For this review, take the finished solid that the model builds, in its own axes (mm). Face numbers are marked on the shaded views. A direction names the side the tool comes from. Round coordinates to 2 decimals unless told otherwise and drop trailing zeros. Write each loop counter-clockwise with the first axis right and the second up, starting at its lowest first coordinate (ties: lowest second). Pieces come first, ordered by that corner, then holes.
from build123d import *

# Parameters (mm, degrees)
SKETCH1_W                  = 30
SKETCH1_H                  = 9.5
CUT_EXTRUDE1_DEPTH         = 3.5
SKETCH3_R                  = 17.4
BOSS_EXTRUDE1_DEPTH        = 4
SKETCH4_R                  = 10
BOSS_EXTRUDE2_DEPTH        = 16
CUT_EXTRUDE2_DEPTH         = 50.759421218
SKETCH6_W                  = 4
SKETCH6_H                  = 26
F_4_CLEARANCE_HOLE1_D      = 3.3
F_2_CLEARANCE_HOLE1_D      = 2.5
F_2_CLEARANCE_HOLE1_DEPTH  = 12
F_2_CLEARANCE_HOLE2_REACH  = 54.582
F_2_CLEARANCE_HOLE2_BORE_R = 1.25
F_2_CLEARANCE_HOLE3_D      = 2.5
F_2_CLEARANCE_HOLE3_DEPTH  = 40
FILLET1_R                  = 3


with BuildPart() as part:
    # Sketch1 → Revolve1 (revolve)
    with BuildSketch(Plane.XZ, mode=Mode.PRIVATE) as revolve1_sk:
        with Locations((15, 5.25)):
            Rectangle(SKETCH1_W, SKETCH1_H)
    revolve(revolve1_sk.sketch.rotate(Axis((0, 0, 10), (0, 0, -1)), 180), axis=Axis((0, 0, 10), (0, 0, -1)))

    # Sketch2 → Cut-Extrude1 (cut)
    with BuildSketch(Plane(origin=(0, 0, 0.5), x_dir=(-1, 0, 0), z_dir=(0, 0, -1))):
        with BuildLine():
            ThreePointArc((1.901854596, -26.932934283), (6.318658968, -26.250229501), (10.562335147, -24.848281153))
            ThreePointArc((10.562335147, -24.848281153), (13.103370267, -25.060195635), (14.379253383, -22.852506912))
            ThreePointArc((14.379253383, -22.852506912), (27, 0), (14.379253383, 22.852506912))
            ThreePointArc((14.379253383, 22.852506912), (13.103370267, 25.060195635), (10.562335147, 24.848281153))
            ThreePointArc((10.562335147, 24.848281153), (6.318658968, 26.250229501), (1.901854596, 26.932934283))
            ThreePointArc((1.901854596, 26.932934283), (0, 27.88125), (-1.901854596, 26.932934283))
            ThreePointArc((-1.901854596, 26.932934283), (-6.318658968, 26.250229501), (-10.562335147, 24.848281153))
            ThreePointArc((-10.562335147, 24.848281153), (-13.103370267, 25.060195635), (-14.379253383, 22.852506912))
            ThreePointArc((-14.379253383, 22.852506912), (-27, 0), (-14.379253383, -22.852506912))
            ThreePointArc((-14.379253383, -22.852506912), (-13.103370267, -25.060195635), (-10.562335147, -24.848281153))
            ThreePointArc((-10.562335147, -24.848281153), (-6.318658968, -26.250229501), (-1.901854596, -26.932934283))
            ThreePointArc((-1.901854596, -26.932934283), (0, -27.88125), (1.901854596, -26.932934283))
        make_face()
    extrude(amount=-CUT_EXTRUDE1_DEPTH, mode=Mode.SUBTRACT)

    # Sketch3 → Boss-Extrude1 (add)
    with BuildSketch(Plane(origin=(0, 0, 4), x_dir=(-1, 0, 0), z_dir=(0, 0, -1))):
        Circle(SKETCH3_R)
    extrude(amount=BOSS_EXTRUDE1_DEPTH)

    # Sketch4 → Boss-Extrude2 (add)
    with BuildSketch(Plane(origin=(0, 0, 0), x_dir=(-1, 0, 0), z_dir=(0, 0, -1))):
        Circle(SKETCH4_R)
    extrude(amount=BOSS_EXTRUDE2_DEPTH)

    # Sketch5 → Cut-Extrude2 (cut, through all)
    with BuildSketch(Plane.XY.offset(10)):
        with BuildLine():
            Line((1, 5), (-1, 5))
            Line((-1, 5), (-1, 3.872983346))
            ThreePointArc((-1, 3.872983346), (0, 4), (1, 3.872983346))
            Line((1, 3.872983346), (1, 5))
        make_face()
    extrude(amount=-CUT_EXTRUDE2_DEPTH, mode=Mode.SUBTRACT)

    # Sketch6 → Cut-Revolve1 (revolve, cut)
    with BuildSketch(Plane.XZ):
        with Locations((2, -3)):
            Rectangle(SKETCH6_W, SKETCH6_H)
    revolve(axis=Axis((0, 0, 10), (0, 0, -1)), mode=Mode.SUBTRACT)

    # #4 Clearance Hole1 (through all)
    with Locations(Plane(origin=(0, 0, 4), x_dir=(-1, 0, 0), z_dir=(0, 0, -1))):
        with Locations((12, -22.95), (0, -25.5), (-12, -22.95), (-12, 22.95), (0, 25.5), (12, 22.95)):
            Hole(F_4_CLEARANCE_HOLE1_D / 2)

    # #2 Clearance Hole1
    with Locations(Plane(origin=(0, 0, -16), x_dir=(-1, 0, 0), z_dir=(0, 0, -1))):
        with Locations((-5.055813485, -5.055813485), (5.055813485, -5.055813485), (5.055813485, 5.055813485), (-5.055813485, 5.055813485)):
            Hole(F_2_CLEARANCE_HOLE1_D / 2, depth=F_2_CLEARANCE_HOLE1_DEPTH)

    # #2 Clearance Hole2 bore (on position points) → #2 Clearance Hole2 (cut, up to next)
    with BuildSketch(Plane(origin=(0, -10, -6.276306458), x_dir=(-1, 0, 0), z_dir=(0, -1, 0)), mode=Mode.PRIVATE) as f_2_clearance_hole2_sk1:
        Circle(F_2_CLEARANCE_HOLE2_BORE_R)
    f_2_clearance_hole2_tool1 = extrude(f_2_clearance_hole2_sk1.sketch, amount=-F_2_CLEARANCE_HOLE2_REACH, mode=Mode.PRIVATE) & part.part
    add(f_2_clearance_hole2_tool1.solids().sort_by_distance((0, -10, -6.276306))[0], mode=Mode.SUBTRACT)

    # #2 Clearance Hole3
    with Locations(Plane(origin=(0, 10, -6.276306458), x_dir=(1, 0, 0), z_dir=(0, 1, 0))):
        with Locations((0, 0)):
            Hole(F_2_CLEARANCE_HOLE3_D / 2, depth=F_2_CLEARANCE_HOLE3_DEPTH)

    # Fillet1
    fillet1_edges = [part.edges().sort_by_distance(p)[0] for p in [
        (10, 0, 0),
    ]]
    fillet(fillet1_edges, radius=FILLET1_R)


solid = part.part
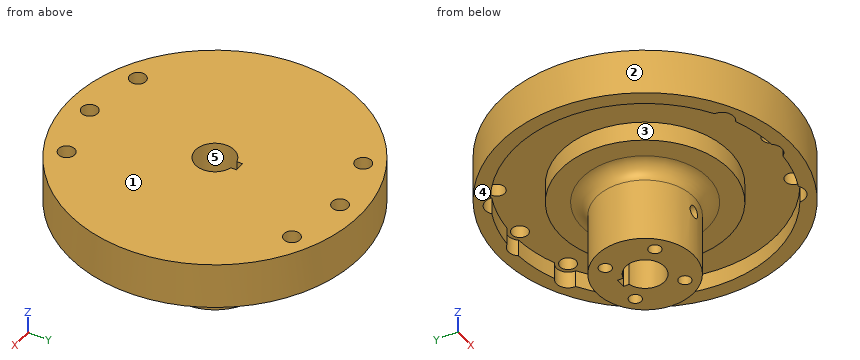
(1) Mouldability with a two-part tool opening along Y and no side actions: class the marked faces 1, 2 and 3 as pulls with the +Y half, pulls with the -Y half, needs draft (parallel to the pull), parting line crosses it, or undercut.
Geometry check:
face 1: needs draft
face 2: parting line crosses it
face 3: undercut
(2) We need section D-D, the plane z = -9. Give the boundary of the cut face in (x, y), and give its area (3 significant figures).
Geometry check:
outline: circle Ø20 at (0, 0); hole circle Ø2.5 at (-5.06, -5.06); hole circle Ø2.5 at (-5.06, 5.06); hole (-1, 3.87) arc R4 ccw (long way) to (1, 3.87) - (1, 5) - (-1, 5) - close; hole circle Ø2.5 at (5.06, -5.06); hole circle Ø2.5 at (5.06, 5.06)
area: 242 mm2
(3) We need section A-A, the plane z = 1.5. Give the boundary of the cut face in (x, y), and give its area (3 significant figures).
Geometry check:
outline: circle Ø60 at (0, 0); circle Ø34.8 at (0, 0); hole (-14.38, -22.85) arc R2.38 ccw to (-10.56, -24.85) arc R27 ccw to (-1.9, -26.93) arc R2.38 ccw to (1.9, -26.93) arc R27 ccw to (10.56, -24.85) arc R2.38 ccw to (14.38, -22.85) arc R27 ccw to (14.38, 22.85) arc R2.38 ccw to (10.56, 24.85) arc R27 ccw to (1.9, 26.93) arc R2.38 ccw to (-1.9, 26.93) arc R27 ccw to (-10.56, 24.85) arc R2.38 ccw to (-14.38, 22.85) arc R27 ccw to start; hole (-1, 3.87) arc R4 ccw (long way) to (1, 3.87) - (1, 5) - (-1, 5) - close
area: 1,420 mm2
(4) For pin 1 Ø7 at (x, y) = (0, 0) entering from -Z; pin 2 Ø0.6 at (y, z) = (4, -12.5) entering from +X; pin 3 Ø2 at (x, z) = (0.5, 2) entering from -Y; pin 4 Ø6 at (x, y) = (13.5, -20.5) entering from -Z, all flat-tipped, find the tip position at first contact; note any pin that passes through.
Geometry check:
pin 1: passes through
pin 2: stops at x = 9.29
pin 3: stops at y = -30
pin 4: stops at z = 0.5
(5) For line 1 along Y through (x, z) = (-12.5, 8.5); line 2 along X through (y, z) = (4.5, -7); line 3 along Y through (x, z) = (-9.5, 2.75), list the stretches that pass through material, from the lowest coordinate up.
Geometry check:
line 1: y = -27.27 to -24.52, -21.38 to 21.38, 24.52 to 27.27
line 2: x = -8.93 to -6.18, -3.94 to -1.02, 1.02 to 3.94, 6.18 to 8.93
line 3: y = -28.46 to -25.27, -14.58 to 14.58, 25.27 to 28.46
(6) We need section C-C, the plane x = 0. State how many separate pieces and enclosed holes the cut face has, and give its area (3 significant figures).
Geometry check:
separate pieces: 6
enclosed holes: 0
area: 537 mm2
(7) For the marked faces 4 and 5, list the 3-axis set-ups (+Z, -Z, +X, -X, +Y, -Y) from which the entire face can be reached by the end or side of a thin tool; tool diameter is ignored.
Geometry check:
face 4: -Z
face 5: +Z, -Z
(8) We need section B-B, the plane y = 0. Give the boundary of the cut face in (x, z).
Geometry check:
outline: (-30, 0.5) - (-27, 0.5) - (-27, 4) - (-17.4, 4) - (-17.4, 0) - (-13, 0) arc R3 cw to (-10, -3) - (-10, -16) - (-4, -16) - (-4, 10) - (-30, 10) - close; (4, -16) - (10, -16) - (10, -3) arc R3 cw to (13, 0) - (17.4, 0) - (17.4, 4) - (27, 4) - (27, 0.5) - (30, 0.5) - (30, 10) - (4, 10) - close
